```python
from build123d import *

# Parameters (mm, degrees)
BOSS_EXTRUDE1_DEPTH                            = 2.54
SKETCH2_R                                      = 2.6
CUT_EXTRUDE1_DEPTH                             = 3.5400001
CUT_EXTRUDE1_DEPTH_BACK                        = 1.0000001
BOSS_EXTRUDE2_DEPTH                            = 2.54
SKETCH5_R                                      = 19.685
CUT_EXTRUDE2_DEPTH                             = 2.54
SKETCH6_W                                      = 56.950712044
SKETCH6_H                                      = 76.2
BOSS_EXTRUDE3_DEPTH                            = 2.54
SKETCH7_W                                      = 56.950712044
SKETCH7_H                                      = 76.2
BOSS_EXTRUDE5_DEPTH                            = 2.54
SKETCH10_W                                     = 56.950712044
SKETCH10_H                                     = 2.54
SKETCH8_W                                      = 56.950712044
SKETCH8_H                                      = 2.54
CUT_EXTRUDE3_REACH                             = 78.2
SKETCH12_R                                     = 4.44110741
CSK_FOR_M5_FLAT_HEAD_MACHINE_SCREW1_AT_2_COUNT = 2
CSK_FOR_M5_FLAT_HEAD_MACHINE_SCREW1_AT_2_PITCH = 38.1
CSK_FOR_M5_FLAT_HEAD_MACHINE_SCREW1_AT_3_COUNT = 2
CSK_FOR_M5_FLAT_HEAD_MACHINE_SCREW1_AT_3_PITCH = 50.8
CSK_FOR_M5_FLAT_HEAD_MACHINE_SCREW1_AT_4_COUNT = 2
CSK_FOR_M5_FLAT_HEAD_MACHINE_SCREW1_AT_4_PITCH = 63.5
CSK_FOR_M5_FLAT_HEAD_MACHINE_SCREW1_AT_5_COUNT = 2
CSK_FOR_M5_FLAT_HEAD_MACHINE_SCREW1_AT_5_PITCH = 88.9
CSK_FOR_M5_FLAT_HEAD_MACHINE_SCREW1_AT_6_COUNT = 2
CSK_FOR_M5_FLAT_HEAD_MACHINE_SCREW1_AT_6_PITCH = 96.720318444
CSK_FOR_M5_FLAT_HEAD_MACHINE_SCREW1_AT_7_COUNT = 2
CSK_FOR_M5_FLAT_HEAD_MACHINE_SCREW1_AT_7_PITCH = 139.7
CSK_FOR_M5_FLAT_HEAD_MACHINE_SCREW1_AT_8_COUNT = 2
CSK_FOR_M5_FLAT_HEAD_MACHINE_SCREW1_AT_8_PITCH = 144.802278988
SKETCH26_R                                     = 3
CUT_EXTRUDE5_DEPTH                             = 10


with BuildPart() as part:
    # Sketch3 → Boss-Extrude1 (new body)
    with BuildSketch(Plane(origin=(0, 0, -4.819), x_dir=(-1, 0, 0), z_dir=(0, 0, -1))):
        with BuildLine():
            Line((28.440509101, 7.854930932), (26.839601475, 7.854930932))
            ThreePointArc((26.839601475, 7.854930932), (22.744771928, 11.949760479), (26.839601475, 16.044590025))
            Line((26.839601475, 16.044590025), (28.440509101, 16.044590025))
            add(Edge.make_bspline(
                [(28.440509101, 16.044590025), (28.459137134, 16.044109711), (28.475836336, 16.060808913), (28.475356022, 16.079436946)],
                knots=[2.356803478, 2.356803478, 2.356803478, 2.356803478, 3.926381829, 3.926381829, 3.926381829, 3.926381829], degree=3))
            Line((28.475356022, 16.079436946), (28.475356022, 25.845))
            ThreePointArc((28.475356022, 25.845), (27.70494258, 27.70494258), (25.845, 28.475356022))
            Line((25.845, 28.475356022), (-7.820084012, 28.475356022))
            add(Edge.make_bspline(
                [(-7.820084012, 28.475356022), (-7.838712044, 28.475836336), (-7.855411247, 28.459137134), (-7.854930932, 28.440509101)],
                knots=[-0.784789176, -0.784789176, -0.784789176, -0.784789176, 0.784789176, 0.784789176, 0.784789176, 0.784789176], degree=3))
            Line((-7.854930932, 28.440509101), (-7.854930932, 26.839601475))
            ThreePointArc((-7.854930932, 26.839601475), (-11.949760479, 22.744771928), (-16.044590025, 26.839601475))
            Line((-16.044590025, 26.839601475), (-16.044590025, 28.440509101))
            add(Edge.make_bspline(
                [(-16.044590025, 28.440509101), (-16.044109711, 28.459137134), (-16.060808913, 28.475836336), (-16.079436946, 28.475356022)],
                knots=[2.356803478, 2.356803478, 2.356803478, 2.356803478, 3.926381829, 3.926381829, 3.926381829, 3.926381829], degree=3))
            Line((-16.079436946, 28.475356022), (-25.845, 28.475356022))
            ThreePointArc((-25.845, 28.475356022), (-27.70494258, 27.70494258), (-28.475356022, 25.845))
            Line((-28.475356022, 25.845), (-28.475356022, -7.820084012))
            add(Edge.make_bspline(
                [(-28.475356022, -7.820084012), (-28.475836336, -7.838712044), (-28.459137134, -7.855411247), (-28.440509101, -7.854930932)],
                knots=[-0.784789176, -0.784789176, -0.784789176, -0.784789176, 0.784789176, 0.784789176, 0.784789176, 0.784789176], degree=3))
            Line((-28.440509101, -7.854930932), (-26.839601475, -7.854930932))
            ThreePointArc((-26.839601475, -7.854930932), (-22.744771928, -11.949760479), (-26.839601475, -16.044590025))
            Line((-26.839601475, -16.044590025), (-28.440509101, -16.044590025))
            add(Edge.make_bspline(
                [(-28.440509101, -16.044590025), (-28.459137134, -16.044109711), (-28.475836336, -16.060808913), (-28.475356022, -16.079436946)],
                knots=[2.356803478, 2.356803478, 2.356803478, 2.356803478, 3.926381829, 3.926381829, 3.926381829, 3.926381829], degree=3))
            Line((-28.475356022, -16.079436946), (-28.475356022, -25.845))
            ThreePointArc((-28.475356022, -25.845), (-27.70494258, -27.70494258), (-25.845, -28.475356022))
            Line((-25.845, -28.475356022), (7.820084012, -28.475356022))
            add(Edge.make_bspline(
                [(7.820084012, -28.475356022), (7.838712044, -28.475836336), (7.855411247, -28.459137134), (7.854930932, -28.440509101)],
                knots=[-0.784789176, -0.784789176, -0.784789176, -0.784789176, 0.784789176, 0.784789176, 0.784789176, 0.784789176], degree=3))
            Line((7.854930932, -28.440509101), (7.854930932, -26.839601475))
            ThreePointArc((7.854930932, -26.839601475), (11.949760479, -22.744771928), (16.044590025, -26.839601475))
            Line((16.044590025, -26.839601475), (16.044590025, -28.440509101))
            add(Edge.make_bspline(
                [(16.044590025, -28.440509101), (16.044109711, -28.459137134), (16.060808913, -28.475836336), (16.079436946, -28.475356022)],
                knots=[2.356803478, 2.356803478, 2.356803478, 2.356803478, 3.926381829, 3.926381829, 3.926381829, 3.926381829], degree=3))
            Line((16.079436946, -28.475356022), (25.845, -28.475356022))
            ThreePointArc((25.845, -28.475356022), (27.70494258, -27.70494258), (28.475356022, -25.845))
            Line((28.475356022, -25.845), (28.475356022, 7.820084012))
            add(Edge.make_bspline(
                [(28.475356022, 7.820084012), (28.475836336, 7.838712044), (28.459137134, 7.855411247), (28.440509101, 7.854930932)],
                knots=[-0.784789176, -0.784789176, -0.784789176, -0.784789176, 0.784789176, 0.784789176, 0.784789176, 0.784789176], degree=3))
        make_face()
    extrude(amount=BOSS_EXTRUDE1_DEPTH)

    # Sketch2 → Cut-Extrude1 (cut, two sides)
    with BuildSketch(Plane(origin=(0, 0, -4.819), x_dir=(-1, 0, 0), z_dir=(0, 0, -1))) as cut_extrude1_sk:
        with Locations((-23.573172318, -23.573172318)):
            Circle(SKETCH2_R)
        with Locations((-23.573172318, 23.573172318)):
            Circle(SKETCH2_R)
        with Locations((23.573172318, 23.573172318)):
            Circle(SKETCH2_R)
        with Locations((23.573172318, -23.573172318)):
            Circle(SKETCH2_R)
    extrude(amount=CUT_EXTRUDE1_DEPTH, mode=Mode.SUBTRACT)
    extrude(cut_extrude1_sk.sketch, amount=-CUT_EXTRUDE1_DEPTH_BACK, mode=Mode.SUBTRACT)

    # Sketch4 → Boss-Extrude2 (add)
    with BuildSketch(Plane.XY.offset(-4.819)):
        with BuildLine():
            Line((-28.475356022, 25.845), (-28.475356022, 79.275356022))
            Line((-28.475356022, 79.275356022), (28.475356022, 79.275356022))
            Line((28.475356022, 79.275356022), (28.475356022, 25.845))
            ThreePointArc((28.475356022, 25.845), (27.70494258, 27.70494258), (25.845, 28.475356022))
            Line((25.845, 28.475356022), (-25.845, 28.475356022))
            ThreePointArc((-25.845, 28.475356022), (-27.70494258, 27.70494258), (-28.475356022, 25.845))
        make_face()
        with BuildLine():
            Line((-28.475356022, -25.845), (-28.475356022, -79.275356022))
            Line((-28.475356022, -79.275356022), (28.475356022, -79.275356022))
            Line((28.475356022, -79.275356022), (28.475356022, -25.845))
            ThreePointArc((28.475356022, -25.845), (27.70494258, -27.70494258), (25.845, -28.475356022))
            Line((25.845, -28.475356022), (-25.845, -28.475356022))
            ThreePointArc((-25.845, -28.475356022), (-27.70494258, -27.70494258), (-28.475356022, -25.845))
        make_face()
    extrude(amount=-BOSS_EXTRUDE2_DEPTH)

    # Sketch5 → Cut-Extrude2 (cut)
    with BuildSketch(Plane.XY.offset(-4.819)):
        Circle(SKETCH5_R)
    extrude(amount=-CUT_EXTRUDE2_DEPTH, mode=Mode.SUBTRACT)

    # Sketch6 → Boss-Extrude3 (add)
    with BuildSketch(Plane(origin=(0, 79.275356022, 0), x_dir=(1, 0, 0), z_dir=(0, 1, 0))):
        with Locations((0, 42.919)):
            Rectangle(SKETCH6_W, SKETCH6_H)
    extrude(amount=BOSS_EXTRUDE3_DEPTH)

    # Sketch7 → Boss-Extrude5 (add)
    with BuildSketch(Plane.XZ.offset(79.275356022)):
        with Locations((0, -42.919)):
            Rectangle(SKETCH7_W, SKETCH7_H)
    extrude(amount=BOSS_EXTRUDE5_DEPTH)

    # Sketch10 → Loft1 section 0
    with BuildSketch(Plane.XZ.offset(-79.275356022)):
        with Locations((0, -79.749)):
            Rectangle(SKETCH10_W, SKETCH10_H)
    # Sketch8 → Loft1 section 1
    with BuildSketch(Plane(origin=(0, -79.275356022, 0), x_dir=(1, 0, 0), z_dir=(0, 1, 0))):
        with Locations((0, 79.749)):
            Rectangle(SKETCH8_W, SKETCH8_H)
    loft()

    # Sketch12 → Cut-Extrude3 (cut, up to next)
    with BuildSketch(Plane.XY.offset(-4.819), mode=Mode.PRIVATE) as cut_extrude3_sk1:
        with Locations((-11.949760479, -26.839601475)):
            Circle(SKETCH12_R)
    cut_extrude3_tool1 = extrude(cut_extrude3_sk1.sketch, amount=-CUT_EXTRUDE3_REACH, mode=Mode.PRIVATE) & part.part
    add(cut_extrude3_tool1.solids().sort_by_distance((-11.94976, -26.839601, -4.819))[0], mode=Mode.SUBTRACT)
    # Sketch12 → Cut-Extrude3 (cut, up to next)
    with BuildSketch(Plane.XY.offset(-4.819), mode=Mode.PRIVATE) as cut_extrude3_sk2:
        with Locations((11.949760479, 26.839601475)):
            Circle(SKETCH12_R)
    cut_extrude3_tool2 = extrude(cut_extrude3_sk2.sketch, amount=-CUT_EXTRUDE3_REACH, mode=Mode.PRIVATE) & part.part
    add(cut_extrude3_tool2.solids().sort_by_distance((11.94976, 26.839601, -4.819))[0], mode=Mode.SUBTRACT)

    # Sketch20 → CSK for M5 Flat Head Machine Screw1 (revolve, cut)
    with BuildSketch(Plane(origin=(-19.05, 69.85, -78.479), x_dir=(0, -1, 0), z_dir=(1, 0, 0))):
        Polygon((0, 0), (0, 2.54), (2.75, 2.54), (2.75, 2.45), (5.2, 0), align=None)
    csk_for_m5_flat_head_machine_screw1 = revolve(axis=Axis((-19.05, 69.85, -72.129), (0, 0, -1)), mode=Mode.SUBTRACT)

    # CSK for M5 Flat Head Machine Screw1 at 2: CSK for M5 Flat Head Machine Screw1 ×2
    with Locations(*[(i * CSK_FOR_M5_FLAT_HEAD_MACHINE_SCREW1_AT_2_PITCH, 0, 0) for i in range(1, CSK_FOR_M5_FLAT_HEAD_MACHINE_SCREW1_AT_2_COUNT)]):
        add(csk_for_m5_flat_head_machine_screw1, mode=Mode.SUBTRACT)

    # CSK for M5 Flat Head Machine Screw1 at 3: CSK for M5 Flat Head Machine Screw1 ×2
    with Locations(*[(0, -i * CSK_FOR_M5_FLAT_HEAD_MACHINE_SCREW1_AT_3_PITCH, 0) for i in range(1, CSK_FOR_M5_FLAT_HEAD_MACHINE_SCREW1_AT_3_COUNT)]):
        add(csk_for_m5_flat_head_machine_screw1, mode=Mode.SUBTRACT)

    # CSK for M5 Flat Head Machine Screw1 at 4: CSK for M5 Flat Head Machine Screw1 ×2
    with Locations(*[Vector(0.6, -0.8, 0) * (i * CSK_FOR_M5_FLAT_HEAD_MACHINE_SCREW1_AT_4_PITCH) for i in range(1, CSK_FOR_M5_FLAT_HEAD_MACHINE_SCREW1_AT_4_COUNT)]):
        add(csk_for_m5_flat_head_machine_screw1, mode=Mode.SUBTRACT)

    # CSK for M5 Flat Head Machine Screw1 at 5: CSK for M5 Flat Head Machine Screw1 ×2
    with Locations(*[(0, -i * CSK_FOR_M5_FLAT_HEAD_MACHINE_SCREW1_AT_5_PITCH, 0) for i in range(1, CSK_FOR_M5_FLAT_HEAD_MACHINE_SCREW1_AT_5_COUNT)]):
        add(csk_for_m5_flat_head_machine_screw1, mode=Mode.SUBTRACT)

    # CSK for M5 Flat Head Machine Screw1 at 6: CSK for M5 Flat Head Machine Screw1 ×2
    with Locations(*[Vector(0.393919299, -0.91914503, 0) * (i * CSK_FOR_M5_FLAT_HEAD_MACHINE_SCREW1_AT_6_PITCH) for i in range(1, CSK_FOR_M5_FLAT_HEAD_MACHINE_SCREW1_AT_6_COUNT)]):
        add(csk_for_m5_flat_head_machine_screw1, mode=Mode.SUBTRACT)

    # CSK for M5 Flat Head Machine Screw1 at 7: CSK for M5 Flat Head Machine Screw1 ×2
    with Locations(*[(0, -i * CSK_FOR_M5_FLAT_HEAD_MACHINE_SCREW1_AT_7_PITCH, 0) for i in range(1, CSK_FOR_M5_FLAT_HEAD_MACHINE_SCREW1_AT_7_COUNT)]):
        add(csk_for_m5_flat_head_machine_screw1, mode=Mode.SUBTRACT)

    # CSK for M5 Flat Head Machine Screw1 at 8: CSK for M5 Flat Head Machine Screw1 ×2
    with Locations(*[Vector(0.263117406, -0.964763821, 0) * (i * CSK_FOR_M5_FLAT_HEAD_MACHINE_SCREW1_AT_8_PITCH) for i in range(1, CSK_FOR_M5_FLAT_HEAD_MACHINE_SCREW1_AT_8_COUNT)]):
        add(csk_for_m5_flat_head_machine_screw1, mode=Mode.SUBTRACT)

    # Sketch26 → Cut-Extrude5 (cut)
    with BuildSketch(Plane.XY.offset(-78.479)):
        with Locations((0, 53.5)):
            Circle(SKETCH26_R)
        with Locations((0, -53.5)):
            Circle(SKETCH26_R)
    extrude(amount=-CUT_EXTRUDE5_DEPTH, mode=Mode.SUBTRACT)


solid = part.part
```
The listing builds one solid part. Answer for the finished solid, in the listing's coordinates (mm). A direction names the side the tool comes from. Coordinates: 2 decimals unless noted, no trailing zeros. Write each loop counter-clockwise with the first axis right and the second up, starting at its lowest first coordinate (ties: lowest second). Pieces come first, ordered by that corner, then holes. Notation, with made-up numbers: (51.25, -20) - (74.25, -20) arc R17 cw to (74.25, -9) - close; hole circle Ø3 at (46.25, 12). An arc over 180 degrees is marked (long way). Return JSON: item names as keys, results as strings. Group by question number.
Q1. Which of the six approach directions +Z, -Z, +X, -X, +Y, -Y give full straight-line access (tool end or side, diameter ignored) to faces 5 (the flat face through (0, -79.275, -42)), 6 (the flat face through (-28.475, 0, -79)), 7 (the conical face through (-19.9, 67.1, -80.8)), 8 (the cylindrical face through (-22.746, 11.86, -6.071)), 9 (the cylindrical face through (-12.528, -22.436, -6.071))?
Q2. Find the intervals of material crossed by line 1 along Y through (x, z) = (-1.5, -26.5); line 2 along Z through (x, y) = (17.5, -44); line 3 along Z through (x, y) = (16, -9), in increasing order. Write a range as [from, to].
Q3. The part is cut by section A-A on x = 0. Write down the section's boundary in (y, z) (3 decimals).
Q4. For a pull along Z with two mould halves and no side action, classify faces 1 (the conical face through (16.171, -69.472, -80.776)), 2 (the conical face through (21.626, -20.39, -80.776)), 3 (the cylindrical face through (-21.51, -25.155, -6.071)), 4 (the flat face through (0, -1, -81.019)) as +Z half, -Z half, draft (parallel to the pull), parting line (faces both ways), or undercut.
Q5. Flat-ended cylindrical pins translate along their axes: pin 1 Ø8 at (x, y) = (11.95, 26.84) entering from +Z; pin 2 Ø3.5 at (x, y) = (-19.05, -69.85) entering from -Z. Find the tip coordinate at first contact, or state that the pin passes through.
Q6. The part is cut by section B-B on y = 47. Write down the section's boundary in (x, z).
Q7. The part is cut by section C-C on z = -63.5. Write down the section's boundary in (x, y).
Q8. The part is cut by section D-D on y = -69.85. Write down the section's boundary in (x, z).
Evaluation:
{
 "1": {"face 5": "+X, -X", "face 6": "+Z, -Z, -X, +Y, -Y", "face 7": "none", "face 8": "+Z, -X", "face 9": "+Z"},
 "2": {"line 1": "y = [-81.82, -79.28], [79.28, 81.82]", "line 2": "z = [-81.02, -78.48], [-7.36, -4.82]", "line 3": "z = [-81.02, -78.48]"},
 "3": {"outline": "(-81.815, -81.019) - (-56.5, -81.019) - (-56.5, -78.479) - (-79.275, -78.479) - (-79.275, -7.359) - (-19.685, -7.359) - (-19.685, -4.819) - (-81.815, -4.819) - close; (-50.5, -81.019) - (50.5, -81.019) - (50.5, -78.479) - (-50.5, -78.479) - close; (19.685, -7.359) - (79.275, -7.359) - (79.275, -78.479) - (56.5, -78.479) - (56.5, -81.019) - (81.815, -81.019) - (81.815, -4.819) - (19.685, -4.819) - close"},
 "4": {"face 1": "undercut", "face 2": "undercut", "face 3": "draft", "face 4": "-Z half"},
 "5": {"pin 1": "stops at z = -78.48", "pin 2": "stops at z = -7.36"},
 "6": {"outline": "(-28.48, -81.02) - (28.48, -81.02) - (28.48, -78.48) - (-28.48, -78.48) - close; (-28.48, -7.36) - (28.48, -7.36) - (28.48, -4.82) - (-28.48, -4.82) - close"},
 "7": {"outline": "(-28.48, -81.82) - (28.48, -81.82) - (28.48, -79.28) - (-28.48, -79.28) - close; (-28.48, 79.28) - (28.48, 79.28) - (28.48, 81.82) - (-28.48, 81.82) - close"},
 "8": {"outline": "(-28.48, -81.02) - (-21.8, -81.02) - (-21.8, -80.93) - (-24.25, -78.48) - (-28.48, -78.48) - close; (-28.48, -7.36) - (28.48, -7.36) - (28.48, -4.82) - (-28.48, -4.82) - close; (-16.3, -81.02) - (16.3, -81.02) - (16.3, -80.93) - (13.85, -78.48) - (-13.85, -78.48) - (-16.3, -80.93) - close; (21.8, -81.02) - (28.48, -81.02) - (28.48, -78.48) - (24.25, -78.48) - (21.8, -80.93) - close"}
}
